from build123d import *

# Parameters (mm, degrees)
F0_R     = 15
F0_R_2   = 16.5
F1_DEPTH = 6
F2_DEPTH = 4
F3_DEPTH = 9


with BuildPart() as f1:
    # F0 (on Top) → F1 (new body)
    with BuildSketch(Plane.XY):
        with BuildLine():
            ThreePointArc((0, -77), (15.556349, -70.556349), (22, -55))
            Line((22, -55), (22, 55))
            ThreePointArc((22, 55), (15.556349, 70.556349), (0, 77))
            ThreePointArc((0, 77), (-15.556349, 70.556349), (-22, 55))
            Line((-22, 55), (-22, -55))
            ThreePointArc((-22, -55), (-15.556349, -70.556349), (0, -77))
        make_face()
        with Locations((0, -45)):
            Circle(F0_R, mode=Mode.SUBTRACT)
        Circle(F0_R_2, mode=Mode.SUBTRACT)
        with Locations((0, 45)):
            Circle(F0_R_2, mode=Mode.SUBTRACT)
        with Locations((0, -45)):
            Circle(F0_R)
        with Locations((0, 45)):
            Circle(F0_R_2)
    extrude(amount=F1_DEPTH)

    # F0 (on Top) → F2 (join)
    with BuildSketch(Plane.XY):
        with Locations((0, -45)):
            Circle(F0_R)
        Circle(F0_R_2)
        with Locations((0, 45)):
            Circle(F0_R_2)
    extrude(amount=F2_DEPTH)

    # F0 (on Top) → F3 (join)
    with BuildSketch(Plane.XY):
        with BuildLine():
            ThreePointArc((0, -80), (17.67767, -72.67767), (25, -55))
            Line((25, -55), (25, 55))
            ThreePointArc((25, 55), (17.67767, 72.67767), (0, 80))
            ThreePointArc((0, 80), (-17.67767, 72.67767), (-25, 55))
            Line((-25, 55), (-25, -55))
            ThreePointArc((-25, -55), (-17.67767, -72.67767), (0, -80))
        make_face()
        with BuildLine():
            Line((22, 55), (22, -55))
            ThreePointArc((22, -55), (15.556349, -70.556349), (0, -77))
            ThreePointArc((0, -77), (-15.556349, -70.556349), (-22, -55))
            Line((-22, -55), (-22, 55))
            ThreePointArc((-22, 55), (-15.556349, 70.556349), (0, 77))
            ThreePointArc((0, 77), (15.556349, 70.556349), (22, 55))
        make_face(mode=Mode.SUBTRACT)
    extrude(amount=F3_DEPTH)


solid = f1.part
Verification items for the finished model (mm, model axes). A direction names the side the tool comes from. Give positions to 0.01 mm unless a question says otherwise; leave off trailing zeros. Order: outer loops, then holes, each group sorted by start corner. A loop starts at its lowest first (then second) coordinate and runs counter-clockwise, first axis right, second up. Notation, with made-up numbers: M 11,67 L 18,67 A29 cw 18,94 Z; hole C 34,47.5 d5. An arc over 180 degrees is marked long. Answer as a JSON object with one key per item and string values. Group by question number.
1) Cross-section at B-B (x = 18). Enter the section's corners in (y, z).
2) Cross-section at D-D (x = 12). Enter the section's corners in (y, z).
3) Cross-section at A-A (y = 0). Enter the section's corners in (x, z), then the cut area to 3 significant figures.
4) Mould release check, pull along Y, two halves, no side actions. Record for faces 1 (the face through (-22.3, 0.4, 9)), 2 (the face through (0, 18, 6)): released by +Y, released by -Y, zero draft, split by the parting line, or undercut.
5) Depth check by flat-ended pin: pin 1 Ø3 at (x, z) = (2.5, 4.5) entering from +Y; pin 2 Ø13 at (x, y) = (-3.5, 36) entering from +Z. Enter the tip coordinate at first touch or a pass-through.
6) Scan lines: line 1 along Y through (x, z) = (0, 4.8); line 2 along Z through (x, y) = (18, -0.5); line 3 along Z through (x, y) = (6.5, -7.5). Record each from-to range of solid material in increasing order. Write a range as [from, to].
7) Access from +Z, -Z, +X, -X, +Y, -Y to the whole of each face (thin tool, end or side, straight path). Record for faces 3 (the face through (-22, -1, 7)), 4 (the face through (-25, 1, 4)).
8) Cross-section at C-C (y = 22). Enter the section's corners in (x, z).
Result sheet:
{
 "1": {"outline": "M -72.35,0 L 72.35,0 L 72.35,9 L 67.65,9 L 67.65,6 L -67.65,6 L -67.65,9 L -72.35,9 Z"},
 "2": {"outline": "M -76.93,0 L 76.93,0 L 76.93,9 L 73.44,9 L 73.44,6 L 11.32,6 L 11.32,4 L -11.32,4 L -11.32,6 L -73.44,6 L -73.44,9 L -76.93,9 Z"},
 "3": {"outline": "M -25,0 L 25,0 L 25,9 L 22,9 L 22,6 L 16.5,6 L 16.5,4 L -16.5,4 L -16.5,6 L -22,6 L -22,9 L -25,9 Z", "area": "252 mm2"},
 "4": {"face 1": "zero draft", "face 2": "undercut"},
 "5": {"pin 1": "stops at y = 79.98", "pin 2": "stops at z = 6"},
 "6": {"line 1": "y = [-80, -16.5], [16.5, 80]", "line 2": "z = [0, 6]", "line 3": "z = [0, 4]"},
 "7": {"face 3": "+Z", "face 4": "+Z, -Z, -X, +Y, -Y"},
 "8": {"outline": "M -25,0 L 25,0 L 25,9 L 22,9 L 22,6 L -22,6 L -22,9 L -25,9 Z"}
}
